```python
from build123d import *

# Parameters (mm, degrees)
BOSS_EXTRUDE1_DEPTH = 3


with BuildPart() as part:
    # Sketch1 → Boss-Extrude1 (new body)
    with BuildSketch(Plane(origin=(0, 0, 0), x_dir=(0, 0, -1), z_dir=(1, 0, 0))):
        with BuildLine():
            Line((-31.05, 0), (-24.75, 0))
            add(Edge.make_bspline(
                [(-18.5, 30), (-21.89992175, 27.622752142), (-23.338614893, 22.064542324), (-24.603317776, 11.688892455), (-24.929004991, 4.971961719), (-24.75, 0)],
                knots=[0, 0, 0, 0, 0.363581561, 0.525534897, 1, 1, 1, 1], degree=3))
            Line((-18.5, 30), (0, 30))
            Line((0, 30), (0, 36))
            Line((0, 36), (-2.95, 36))
            Line((-2.95, 36), (-2.95, 39))
            ThreePointArc((-2.95, 39), (-23.791917434, 31.05229513), (-34.05, 11.24514296))
            Line((-34.05, 11.24514296), (-34.05, 0))
            Line((-34.05, 0), (-31.05, 0))
        make_face()
        with BuildLine():
            add(Edge.make_bspline(
                [(18.5, 30), (21.89992175, 27.622752142), (23.338614893, 22.064542324), (24.603317776, 11.688892455), (24.929004991, 4.971961719), (24.75, 0)],
                knots=[0, 0, 0, 0, 0.363581561, 0.525534897, 1, 1, 1, 1], degree=3))
            Line((24.75, 0), (31.05, 0))
            Line((31.05, 0), (34.05, 0))
            Line((34.05, 0), (34.05, 11.24514296))
            ThreePointArc((34.05, 11.24514296), (23.791917434, 31.05229513), (2.95, 39))
            Line((2.95, 39), (2.95, 36))
            Line((2.95, 36), (0, 36))
            Line((0, 36), (0, 30))
            Line((0, 30), (18.5, 30))
        make_face()
        Polygon((24.75, 0), (0, 0), (0, -6.3), (24.95, -6.3), (24.95, -41.7), (34.05, -41.7), (34.05, -37.3), (31.05, -37.3), (31.05, 0), align=None)
        Polygon((0, 0), (-24.75, 0), (-31.05, 0), (-31.05, -37.3), (-34.05, -37.3), (-34.05, -41.7), (-24.95, -41.7), (-24.95, -6.3), (0, -6.3), align=None)
    extrude(amount=BOSS_EXTRUDE1_DEPTH)


solid = part.part
```
The model under review builds one solid part; all positions refer to its coordinate system, in mm. A direction names the side the tool comes from. Round coordinates to 2 decimals unless told otherwise and drop trailing zeros. Loops run counter-clockwise (first coordinate to the right, second up) from the corner with the lowest first, then second, coordinate; pieces in that order, holes last. Notation, with made-up numbers: M 82,26.25 L 91,26.25 A7 ccw 91,37.25 Z; hole C -38,-15.75 d1. An arc over 180 degrees is marked long. Write item = value, one per line.
Item 1: Take a section at A-A on y = -27. Write out the cut boundary in (x, z), then the cut area to 3 significant figures.
Return value:
outline = M 0,-31.05 L 3,-31.05 L 3,-24.95 L 0,-24.95 Z; M 0,24.95 L 3,24.95 L 3,31.05 L 0,31.05 Z
area = 36.6 mm2
Item 2: Take a section at C-C on z = -29.5. Write out the cut boundary in (x, y).
Return value:
outline = M 0,-41.7 L 3,-41.7 L 3,24.28 L 0,24.28 Z
Item 3: Take a section at D-D on y = 31. Write out the cut boundary in (x, z).
Return value:
outline = M 0,-23.85 L 3,-23.85 L 3,23.85 L 0,23.85 Z
Item 4: For line 1 (Z direction, x = 1.5, y = -19); line 2 (Z direction, x = 1.2, y = 6); line 3 (Y direction, x = 2.65, z = 6), list the stretches that pass through material, from the lowest coordinate up. Write a range as [from, to].
Return value:
line_1 = [-31.05, -24.95], [24.95, 31.05]
line_2 = [-34.05, -24.77], [24.77, 34.05]
line_3 = [-6.3, 0], [30, 38.85]
Item 5: Insertion check: P1, Ø1.5, axis at x = 1.5, y = -20, coming from the -Z side; P2, Ø0.9, axis at x = 2, z = -1.5, coming from the +Y side; P3, Ø0.9, axis at x = 2, y = -24, coming from the +Z side. Each pin has a flat end and moves straight along its axis. Give the tip position at first contact, or say it passes through.
Return value:
P1 = -31.05
P2 = 36
P3 = 31.05
Item 6: Take a section at B-B on z = -16. Write out the cut boundary in (x, y), then the cut area to 3 significant figures.
Return value:
outline = M 0,-6.3 L 3,-6.3 L 3,0 L 0,0 Z; M 0,30 L 3,30 L 3,36.15 L 0,36.15 Z
area = 37.3 mm2
Item 7: The part is to be moulded in two halves that separate along Z. For faces 1 (the flat face through (1, 36, 0)), 2 (the flat face through (3, -1, 0)), 3 (the flat face through (1, 6, -34.05)), say which applies: released by +Z, released by -Z, zero draft, split by the parting line, or undercut.
Return value:
face_1 = undercut
face_2 = zero draft
face_3 = released by -Z
Item 8: Machinability: for faces 4 (the flat face through (1, 30, 0)), 5 (the flat face through (1, -6.3, 0)), 6 (the flat face through (1, -18, 31.05)), 7 (the flat face through (1, 37, 2.95)), 8 (the flat face through (1, -37.3, -33)), which of the approach directions +Z, -Z, +X, -X, +Y, -Y give a long, thin tool a straight path to every point of the face, cutting with its end or side? Answer none if there is none.
Return value:
face_4 = +X, -X
face_5 = +X, -X, -Y
face_6 = +Z, +X, -X
face_7 = +X, -X, +Y
face_8 = -Z, +X, -X
